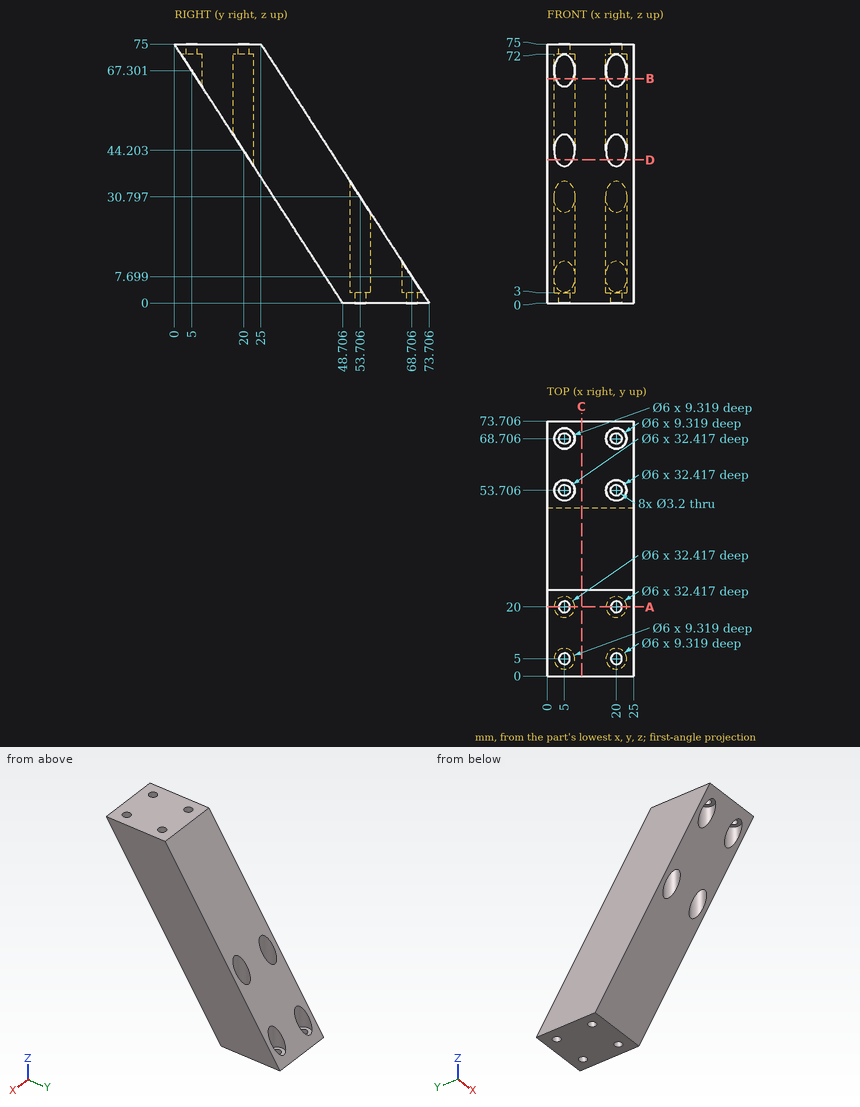
Input: dimensioned drawing with shaded views. Units: mm. Origin: part minimum x, y, z. Coordinates: 2 decimals unless noted, no trailing zeros. Loops run counter-clockwise (first coordinate to the right, second up) from the corner with the lowest first, then second, coordinate; pieces in that order, holes last. Notation, with made-up numbers: (8, 68.5) - (54, 68.5) arc R11 cw to (54, 75.5) - close; hole circle Ø2 at (77.25, 74.25). An arc over 180 degrees is marked (long way). One line per question, with ' | ' between items. Start each with the question number.
(1) First-contact query: pin 1 (5 mm diameter, centred on x = 19, y = 68.5, fed in from +Z); pin 2 (1.8 mm diameter, centred on x = 4.5, y = 70, fed in from +Z); pin 3 (9.5 mm diameter, centred on x = 20, y = 20, fed in from -Z); pin 4 (2.5 mm diameter, centred on x = 5, y = 20, fed in from -Z). Flat tips, straight axial feed; report the tip coordinate or a pass-through.
(2) Cut plane C-C on x = 10. Output: boundary loops of the cut face in (y, z) (1 decimal).
(3) Cut plane B-B on z = 65. Output: boundary loops of the cut face in (x, y), and give its area (3 significant figures).
(4) Cut plane A-A on y = 20. Output: boundary loops of the cut face in (x, z), and give its area (3 significant figures).
(5) Ray query, L1, parallel to X at y = 21.5, z = 44; L2, parallel to Y at x = 17.25, z = 49 (1 decimal); L3, parallel to Z at x = 17.75, y = 8. Return the intervals inside material, ascending. Write a range as from..to.
(6) Cut plane D-D on z = 41.5. Output: boundary loops of the cut face in (x, y) (1 decimal).
Here are the results:
1) pin 1: z = 11.83 | pin 2: z = 3 | pin 3: z = 36.89 | pin 4: through
2) outline: (0, 75) - (48.7, 0) - (73.7, 0) - (25, 75) - close
3) outline: (0, 6.49) - (2.4, 6.49) arc R3 cw to (7.6, 6.49) - (17.4, 6.49) arc R3 cw to (22.6, 6.49) - (25, 6.49) - (25, 31.49) - (0, 31.49) - close; hole circle Ø6 at (5, 20); hole circle Ø6 at (20, 20) | area: 557 mm²
4) outline: (0, 44.2) - (2, 44.2) - (2, 72) - (3.4, 72) - (3.4, 75) - (0, 75) - close; (6.6, 72) - (8, 72) - (8, 44.2) - (17, 44.2) - (17, 72) - (18.4, 72) - (18.4, 75) - (6.6, 75) - close; (21.6, 72) - (23, 72) - (23, 44.2) - (25, 44.2) - (25, 75) - (21.6, 75) - close | area: 417 mm²
5) L1: 0..2.4, 7.6..17.4, 22.6..25 | L2: 16.9..18.8, 21.2..41.9 | L3: 62.68..75
6) outline: (0, 21.8) - (2.6, 21.8) arc R3 cw to (7.4, 21.8) - (17.6, 21.8) arc R3 cw to (22.4, 21.8) - (25, 21.8) - (25, 46.8) - (0, 46.8) - close
